Input: part model. Units: mm. Frame: model coordinates. Face numbers are marked on the shaded views. A direction names the side the tool comes from. Coordinates: 2 decimals unless noted, no trailing zeros. Loops run counter-clockwise (first coordinate to the right, second up) from the corner with the lowest first, then second, coordinate; pieces in that order, holes last. Notation, with made-up numbers: (19.25, -5) - (47.25, -5) arc R19 cw to (47.25, 18) - close; hole circle Ø5 at (58, 47.25). An arc over 180 degrees is marked (long way). Use one line per item in the form item = value.
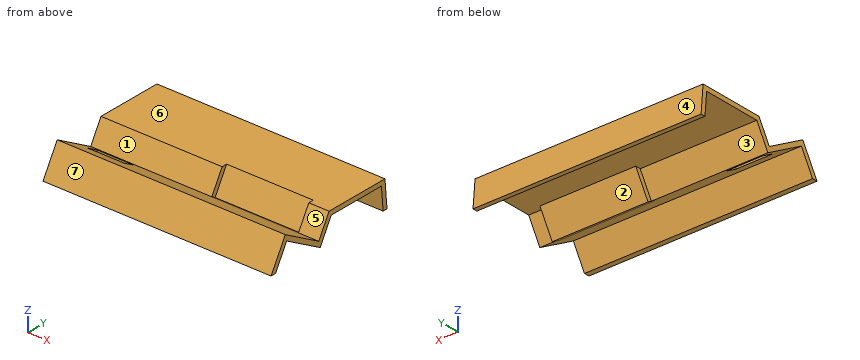
from build123d import *

# Parameters (mm, degrees)
F1_DEPTH = 50
F2_W     = 38
F2_H     = 2
F3_DEPTH = 26.3255735195
F4_T     = -2
F5_W     = 16
F5_H     = 5
F6_DEPTH = 12.7330508076


with BuildPart() as f1:
    # F0 (on Right) → F1 (new body, symmetric)
    with BuildSketch(Plane.YZ):
        Polygon((-22.6491470389, 12.7320508076), (-30, 0), (30, 0), (28.9501360377, 12), (0.0222139979, 12), (-5.3286389632, 2.7320508076), align=None)
    extrude(amount=F1_DEPTH, both=True)

    # F2 (on face) → F3 (cut, through all)
    with BuildSketch(Plane(origin=(0, -0.1491470389, -0.2583302492), x_dir=(1, 0, 0), z_dir=(0, 0.5, 0.8660254038))):
        with Locations((22.1086753011, -4.9807621135)):
            Rectangle(F2_W, F2_H)
    extrude(amount=F3_DEPTH, mode=Mode.SUBTRACT)

    # F4
    f4_openings = [f1.faces().sort_by_distance(p)[0] for p in [
        (0, 0, 0),
        (50, 3.195409, 5.336498),
        (-50, 3.195409, 5.336498),
    ]]
    offset(amount=F4_T, openings=f4_openings, kind=Kind.INTERSECTION)

    # F5 (on Top) → F6 (cut, through all)
    with BuildSketch(Plane.XY):
        with Locations((-37.7319419413, -9.4969761558)):
            Rectangle(F5_W, F5_H)
    extrude(amount=F6_DEPTH, mode=Mode.SUBTRACT)


solid = f1.part
Q1. Set-up query: the marked faces 1, 2 and 3. Return all of +Z, -Z, +X, -X, +Y, -Y with unobstructed straight access to the full face (end or side cutting, diameter ignored); none if empty.
Check values:
face_1 = +Z, +X, -X
face_2 = -Z, +X, -X
face_3 = -Z, -X
Q2. Ray query, line 1 along Y through (x, z) = (37, 1); line 2 along Y through (x, z) = (-29, 1); line 3 along Y through (x, z) = (36, 6). Return the intervals inside material, ascending. Write a range as [from, to].
Check values:
line_1 = [-29.42, -27.11], [-6.33, -1.71], [27.9, 29.91]
line_2 = [-29.42, -27.11], [-6.33, -4.02], [27.9, 29.91]
line_3 = [-26.54, -24.23], [-14.99, -10.99], [-1.13, 1.18], [27.47, 29.48]
Q3. Cut plane D-D, the plane y = 8.5. Return loops of the section in (x, z), then the cut area to 3 significant figures.
Check values:
outline = (-50, 10) - (50, 10) - (50, 12) - (-50, 12) - close
area = 200 mm²
Q4. Cut plane A-A, the plane x = -33. Return loops of the section in (y, z).
Check values:
outline = (-30, 0) - (-27.69, 0) - (-21.92, 10) - (-12, 4.27) - (-12, 6.58) - (-22.65, 12.73) - close; (-7, 1.39) - (-4.6, 0) - (1.18, 10) - (27.12, 10) - (27.99, 0) - (30, 0) - (28.95, 12) - (0.02, 12) - (-5.33, 2.73) - (-7, 3.7) - close
Q5. Cut plane B-B, the plane z = 8. Return loops of the section in (x, y).
Check values:
outline = (-50, -25.38) - (50, -25.38) - (50, -23.07) - (-50, -23.07) - close; (-50, -18.45) - (50, -18.45) - (50, -14.45) - (-50, -14.45) - close; (-50, -2.29) - (3.11, -2.29) - (3.11, 0.02) - (41.11, 0.02) - (41.11, -2.29) - (50, -2.29) - (50, 0.02) - (43.11, 0.02) - (43.11, 2.33) - (1.11, 2.33) - (1.11, 0.02) - (-50, 0.02) - close; (-50, 27.29) - (50, 27.29) - (50, 29.3) - (-50, 29.3) - close
Q6. First-contact query: P1, Ø1.5, axis at x = 14.5, y = 0.5, coming from the +Z side; P2, Ø1.8, axis at x = 14, y = -29, coming from the -Z side; P3, Ø4, axis at x = 25, z = 11, coming from the +Y side. Flat tips, straight axial feed; report the tip coordinate or a pass-through.
Check values:
P1 = 10.13
P2 = 0
P3 = 29.21
Q7. Cut plane C-C, the plane x = -9. Return loops of the section in (y, z), then the cut area to 3 significant figures.
Check values:
outline = (-30, 0) - (-27.69, 0) - (-21.92, 10) - (-4.6, 0) - (1.18, 10) - (27.12, 10) - (27.99, 0) - (30, 0) - (28.95, 12) - (0.02, 12) - (-5.33, 2.73) - (-22.65, 12.73) - close
area = 165 mm²
Q8. Pull-direction query (Y, two-part tool) for the marked faces 4, 5, 6 and 7; classes: pulls with the +Y half, pulls with the -Y half, needs draft (parallel to the pull), parting line crosses it, or undercut.
Check values:
face_4 = pulls with the +Y half
face_5 = undercut
face_6 = needs draft
face_7 = pulls with the -Y half
